Check sheet for the modelled part. Datum: model origin and axes. Units: mm. Give positions to 0.01 mm unless a question says otherwise; leave off trailing zeros. Write each loop counter-clockwise with the first axis right and the second up, starting at its lowest first coordinate (ties: lowest second). Pieces come first, ordered by that corner, then holes. Notation, with made-up numbers: (85.25, 51) -> (121.25, 51) arc R26 ccw to (121.25, 89) -> close; hole circle Ø3 at (74.5, 72). An arc over 180 degrees is marked (long way). Answer as a JSON object with one key per item and string values.
from build123d import *

# Parameters (mm, degrees)
SKETCH1_R           = 2.4638
BOSS_EXTRUDE1_DEPTH = 3.175
SKETCH2_R           = 2.159
CUT_EXTRUDE1_DEPTH  = 159.781746826
SKETCH5_R           = 3.175
SKETCH5_R_2         = 12.7
SKETCH5_R_3         = 2.159
SKETCH5_R_4         = 1.4478
CUT_EXTRUDE2_DEPTH  = 159.781746826
SKETCH6_R           = 2.159
CUT_EXTRUDE3_DEPTH  = 159.781746826
SKETCH5_3_R         = 2.9083
CUT_EXTRUDE4_DEPTH  = 159.781746826
SKETCH5_4_R         = 1.5875
SKETCH5_4_R_2       = 4.7625
CUT_EXTRUDE5_DEPTH  = 159.781746826
SKETCH5_5_R         = 1.5875
CUT_EXTRUDE6_DEPTH  = 2.54
SKETCH5_6_R         = 1.5875
CUT_EXTRUDE7_DEPTH  = 159.781746826


with BuildPart() as part:
    # Sketch1 → Boss-Extrude1 (new body)
    with BuildSketch(Plane.XY):
        Polygon((-111.686526805, -95.25), (-127, -83.918625912), (-127, 83.918625912), (-111.686526805, 95.25), (111.686526805, 95.25), (127, 83.918625912), (127, -83.918625912), (111.686526805, -95.25), align=None)
        with Locations((-95.147512794, 56.885632681)):
            Circle(SKETCH1_R, mode=Mode.SUBTRACT)
        with Locations((-110.256011578, 77.303596941)):
            Circle(SKETCH1_R, mode=Mode.SUBTRACT)
        with Locations(Location((110.256011578, 77.303596941, 0), (0, 0, 180))):
            Circle(SKETCH1_R, mode=Mode.SUBTRACT)
        with Locations(Location((95.147512794, 56.885632681, 0), (0, 0, 180))):
            Circle(SKETCH1_R, mode=Mode.SUBTRACT)
        with Locations(Location((-110.256011578, -77.303596941, 0), (0, 0, 180))):
            Circle(SKETCH1_R, mode=Mode.SUBTRACT)
        with Locations(Location((-95.147512794, -56.885632681, 0), (0, 0, 180))):
            Circle(SKETCH1_R, mode=Mode.SUBTRACT)
        with Locations((110.256011578, -77.303596941)):
            Circle(SKETCH1_R, mode=Mode.SUBTRACT)
        with Locations((95.147512794, -56.885632681)):
            Circle(SKETCH1_R, mode=Mode.SUBTRACT)
    extrude(amount=BOSS_EXTRUDE1_DEPTH)

    # Sketch2 → Cut-Extrude1 (cut, through all)
    with BuildSketch(Plane.XY.offset(3.175)):
        with Locations((42.8625, -58.7375)):
            Circle(SKETCH2_R)
        with Locations((71.4375, -58.7375)):
            Circle(SKETCH2_R)
        with Locations((71.4375, 58.7375)):
            Circle(SKETCH2_R)
        with Locations((42.8625, 58.7375)):
            Circle(SKETCH2_R)
    extrude(amount=-CUT_EXTRUDE1_DEPTH, mode=Mode.SUBTRACT)

    # Sketch5 → Cut-Extrude2 (cut, through all)
    with BuildSketch(Plane(origin=(0, 0, 0), x_dir=(-1, 0, 0), z_dir=(0, 0, -1))):
        with Locations((80.594630637, 48.58004)):
            Circle(SKETCH5_R)
        with Locations((-57.15, 71.4375)):
            Circle(SKETCH5_R_2)
        with Locations((59.995230637, 39.49954)):
            Circle(SKETCH5_R_3)
        with Locations((101.994130637, 39.49954)):
            Circle(SKETCH5_R_3)
        with Locations((59.995230637, -39.49954)):
            Circle(SKETCH5_R_3)
        with Locations((101.994130637, -39.49954)):
            Circle(SKETCH5_R_3)
        with Locations((56.219708857, 15.03413)):
            Circle(SKETCH5_R_4)
        with Locations((56.219708857, -15.03413)):
            Circle(SKETCH5_R_4)
        with Locations((85.937708857, -15.03413)):
            Circle(SKETCH5_R_4)
        with Locations((85.937708857, 15.03413)):
            Circle(SKETCH5_R_4)
        with BuildLine():
            Line((-25.4, 25.4), (-25.4, -25.4))
            ThreePointArc((-25.4, -25.4), (-28.575, -28.575), (-31.75, -25.4))
            Line((-31.75, -25.4), (-31.75, 25.4))
            ThreePointArc((-31.75, 25.4), (-28.575, 28.575), (-25.4, 25.4))
        make_face()
        with BuildLine():
            Line((25.4, 25.4), (25.4, -25.4))
            ThreePointArc((25.4, -25.4), (28.575, -28.575), (31.75, -25.4))
            Line((31.75, -25.4), (31.75, 25.4))
            ThreePointArc((31.75, 25.4), (28.575, 28.575), (25.4, 25.4))
        make_face()
    extrude(amount=-CUT_EXTRUDE2_DEPTH, mode=Mode.SUBTRACT)

    # Sketch6 → Cut-Extrude3 (cut, through all)
    with BuildSketch(Plane(origin=(0, 0, 0), x_dir=(-1, 0, 0), z_dir=(0, 0, -1))):
        with Locations((-76.2, -85.725)):
            Circle(SKETCH6_R)
        with Locations((-25.4, -85.725)):
            Circle(SKETCH6_R)
        with Locations((25.4, -85.725)):
            Circle(SKETCH6_R)
        with Locations((76.2, -85.725)):
            Circle(SKETCH6_R)
        with Locations(Location((76.2, 85.725, 0), (0, 0, 180))):
            Circle(SKETCH6_R)
        with Locations(Location((25.4, 85.725, 0), (0, 0, 180))):
            Circle(SKETCH6_R)
        with Locations(Location((-25.4, 85.725, 0), (0, 0, 180))):
            Circle(SKETCH6_R)
        with Locations(Location((-76.2, 85.725, 0), (0, 0, 180))):
            Circle(SKETCH6_R)
        with Locations((117.475, -25.4)):
            Circle(SKETCH6_R)
        with Locations(Location((117.475, 25.4, 0), (0, 0, 180))):
            Circle(SKETCH6_R)
        with Locations((-117.475, 25.4)):
            Circle(SKETCH6_R)
        with Locations(Location((-117.475, -25.4, 0), (0, 0, 180))):
            Circle(SKETCH6_R)
    extrude(amount=-CUT_EXTRUDE3_DEPTH, mode=Mode.SUBTRACT)

    # Sketch5_3 → Cut-Extrude4 (cut, through all)
    with BuildSketch(Plane(origin=(0, 0, 0), x_dir=(-1, 0, 0), z_dir=(0, 0, -1))):
        with Locations((-42.5, 17.2)):
            Circle(SKETCH5_3_R)
        with Locations(Location((-42.5, -17.2, 0), (0, 0, 180))):
            Circle(SKETCH5_3_R)
        with Locations((42.5, -17.2)):
            Circle(SKETCH5_3_R)
        with Locations(Location((42.5, 17.2, 0), (0, 0, 180))):
            Circle(SKETCH5_3_R)
    extrude(amount=-CUT_EXTRUDE4_DEPTH, mode=Mode.SUBTRACT)

    # Sketch5_4 → Cut-Extrude5 (cut, through all)
    with BuildSketch(Plane(origin=(0, 0, 0), x_dir=(-1, 0, 0), z_dir=(0, 0, -1))):
        with Locations(Location((61.544630637, -54.61, 0), (0, 0, 180))):
            Circle(SKETCH5_4_R)
        with Locations((61.544630637, -67.31)):
            Circle(SKETCH5_4_R)
        with Locations((61.544630637, 54.61)):
            Circle(SKETCH5_4_R)
        with Locations((61.544630637, -80.01)):
            Circle(SKETCH5_4_R)
        with Locations((-50.215369363, -67.31)):
            Circle(SKETCH5_4_R_2)
        with Locations(Location((50.215369363, -67.31, 0), (0, 0, 180))):
            Circle(SKETCH5_4_R_2)
        with Locations(Location((61.544630637, 67.31, 0), (0, 0, 180))):
            Circle(SKETCH5_4_R)
        with Locations(Location((61.544630637, 80.01, 0), (0, 0, 180))):
            Circle(SKETCH5_4_R)
        with Locations((50.215369363, 67.31)):
            Circle(SKETCH5_4_R_2)
    extrude(amount=-CUT_EXTRUDE5_DEPTH, mode=Mode.SUBTRACT)

    # Sketch5_5 → Cut-Extrude6 (cut)
    with BuildSketch(Plane(origin=(0, 0, 0), x_dir=(-1, 0, 0), z_dir=(0, 0, -1))):
        with Locations((38.886108088, 67.31)):
            Circle(SKETCH5_5_R)
        with Locations(Location((38.886108088, 54.61, 0), (0, 0, 180))):
            Circle(SKETCH5_5_R)
        with Locations(Location((38.886108088, -67.31, 0), (0, 0, 180))):
            Circle(SKETCH5_5_R)
    extrude(amount=-CUT_EXTRUDE6_DEPTH, mode=Mode.SUBTRACT)

    # Sketch5_6 → Cut-Extrude7 (cut, through all)
    with BuildSketch(Plane(origin=(0, 0, 0), x_dir=(-1, 0, 0), z_dir=(0, 0, -1))):
        with Locations((38.886108088, 67.31)):
            Circle(SKETCH5_6_R)
        with Locations(Location((38.886108088, 54.61, 0), (0, 0, 180))):
            Circle(SKETCH5_6_R)
        with Locations(Location((38.886108088, -67.31, 0), (0, 0, 180))):
            Circle(SKETCH5_6_R)
    extrude(amount=-CUT_EXTRUDE7_DEPTH, mode=Mode.SUBTRACT)


solid = part.part
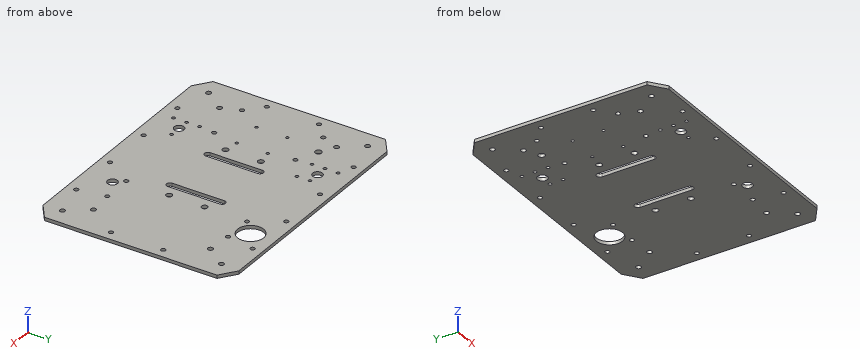
1. Sectioned sample at A-A, the plane y = 9. Enter the section's corners in (x, z) (3 decimals), plus the area to 3 significant figures.
Determined:
{"outline": "(-127, 0) -> (-31.75, 0) -> (-31.75, 3.175) -> (-127, 3.175) -> close; (-25.4, 0) -> (25.4, 0) -> (25.4, 3.175) -> (-25.4, 3.175) -> close; (31.75, 0) -> (127, 0) -> (127, 3.175) -> (31.75, 3.175) -> close", "area": "766 mm^2"}
2. Scan lines: L1, parallel to X at y = -5, z = 3; L2, parallel to X at y = -25, z = 2.9; L3, parallel to X at y = 49, z = 2.35. Record each from-to range of solid material in increasing order. Write a range as [from, to].
Determined:
{"L1": "[-127, -31.75], [-25.4, 25.4], [31.75, 127]", "L2": "[-127, -119.6], [-115.35, -31.75], [-25.4, 25.4], [31.75, 115.35], [119.6, 127]", "L3": "[-127, -83.74], [-77.45, 127]"}
3. Go/stop test with flat-tipped pins: P1, Ø5.5, axis at x = 42.86, y = -58.74, coming from the -Z side; P2, Ø1.9, axis at x = -61.54, y = 80.01, coming from the -Z side. Record where each tip stops, or that it passes through.
Determined:
{"P1": "z = 0", "P2": "through"}
4. Sectioned sample at B-B, the plane z = 1.3. State how many separate pieces and enclosed holes the cut face has, plus the area to 3 significant figures.
Determined:
{"separate pieces": "1", "enclosed holes": "52", "area": "45,900 mm^2"}
